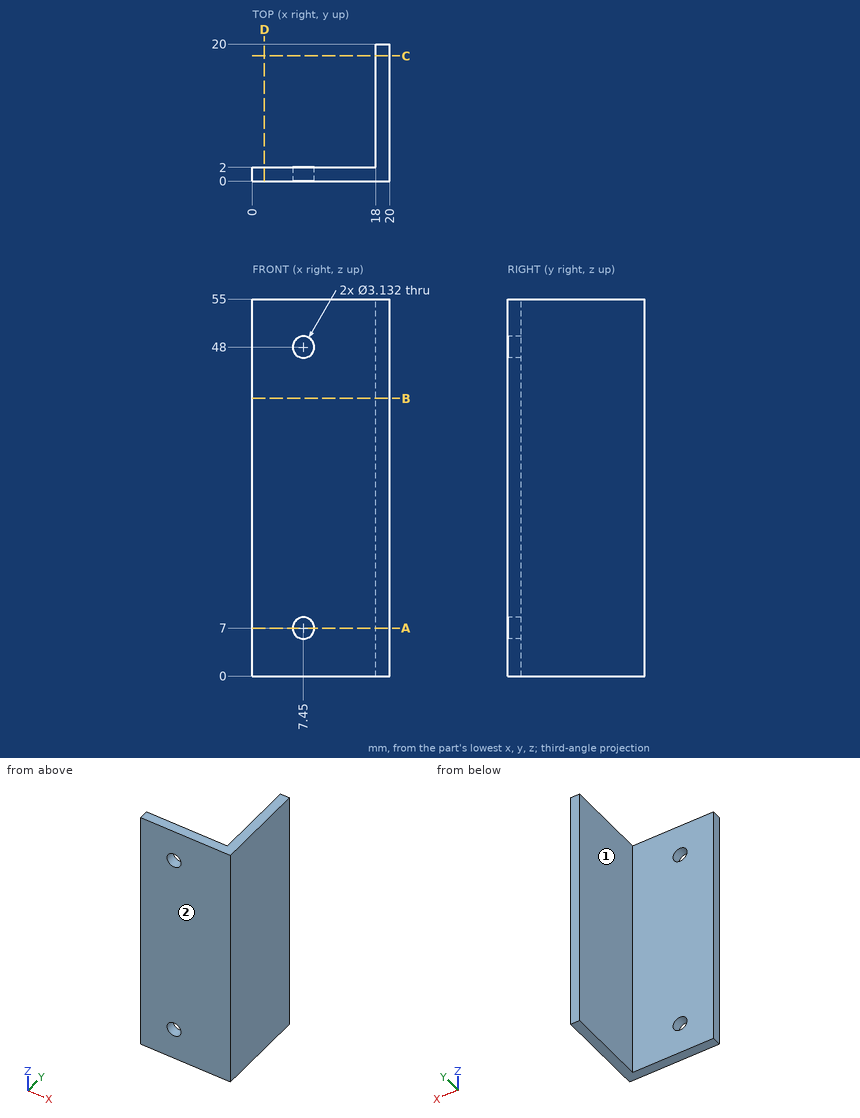
Could you check a few things on this drawing? It's one solid part, dimensions in mm from its lowest x, y, z. A direction names the side the tool comes from. Round coordinates to 2 decimals unless told otherwise and drop trailing zeros. Loops run counter-clockwise (first coordinate to the right, second up) from the corner with the lowest first, then second, coordinate; pieces in that order, holes last. Notation, with made-up numbers: (1.25, -36.5) -> (49.25, -36.5) arc R10 cw to (49.25, -28.5) -> close; hole circle Ø10 at (43.25, -7). An arc over 180 degrees is marked (long way). One line per item, written item: value. Start each with the question number.
1. For the marked faces 1 and 2, which set-ups out of +Z, -Z, +X, -X, +Y, -Y let a thin tool reach every point of the face, with its end or its side?
2. If I drill on probe 1 along X at (y, z) = (14.75, 22.5); probe 2 along Y at (x, z) = (16.75, 8); probe 3 along Z at (x, y) = (6.75, 1.75), over which ranges is the centre line in solid material (lowest first)?
3. If we section it at B-B, the plane z = 40.5: Write out the boundary of the cut face in (x, y).
4. If we section it at D-D, the plane x = 1.75: Write out the boundary of the cut face in (y, z), then the cut area to 3 significant figures.
5. If we section it at A-A, the plane z = 7: Write out the boundary of the cut face in (x, y).
6. If we section it at C-C, the plane y = 18.25: Write out the boundary of the cut face in (x, z).
7. For pin 1 (3 mm diameter, centred on x = 7.45, z = 7, fed in from +Y); pin 2 (1 mm diameter, centred on x = 5, z = 26.5, fed in from +Y); pin 3 (3 mm diameter, centred on y = 18, z = 43, fed in from -X), each with a flat end and sliding along its axis, tell me the tip position at first contact or that it passes through.
Calculated:
1. face 1: +Z, -Z, -X, +Y
1. face 2: +Z, -Z, +X, -X, -Y
2. probe 1: x = 18 to 20
2. probe 2: y = 0 to 2
2. probe 3: z = 0 to 5.6, 8.4 to 46.6, 49.4 to 55
3. outline: (0, 0) -> (20, 0) -> (20, 20) -> (18, 20) -> (18, 2) -> (0, 2) -> close
4. outline: (0, 0) -> (2, 0) -> (2, 55) -> (0, 55) -> close
4. area: 110 mm²
5. outline: (0, 0) -> (5.88, 0) -> (5.88, 2) -> (0, 2) -> close; (9.02, 0) -> (20, 0) -> (20, 20) -> (18, 20) -> (18, 2) -> (9.02, 2) -> close
6. outline: (18, 0) -> (20, 0) -> (20, 55) -> (18, 55) -> close
7. pin 1: passes through
7. pin 2: stops at y = 2
7. pin 3: stops at x = 18
